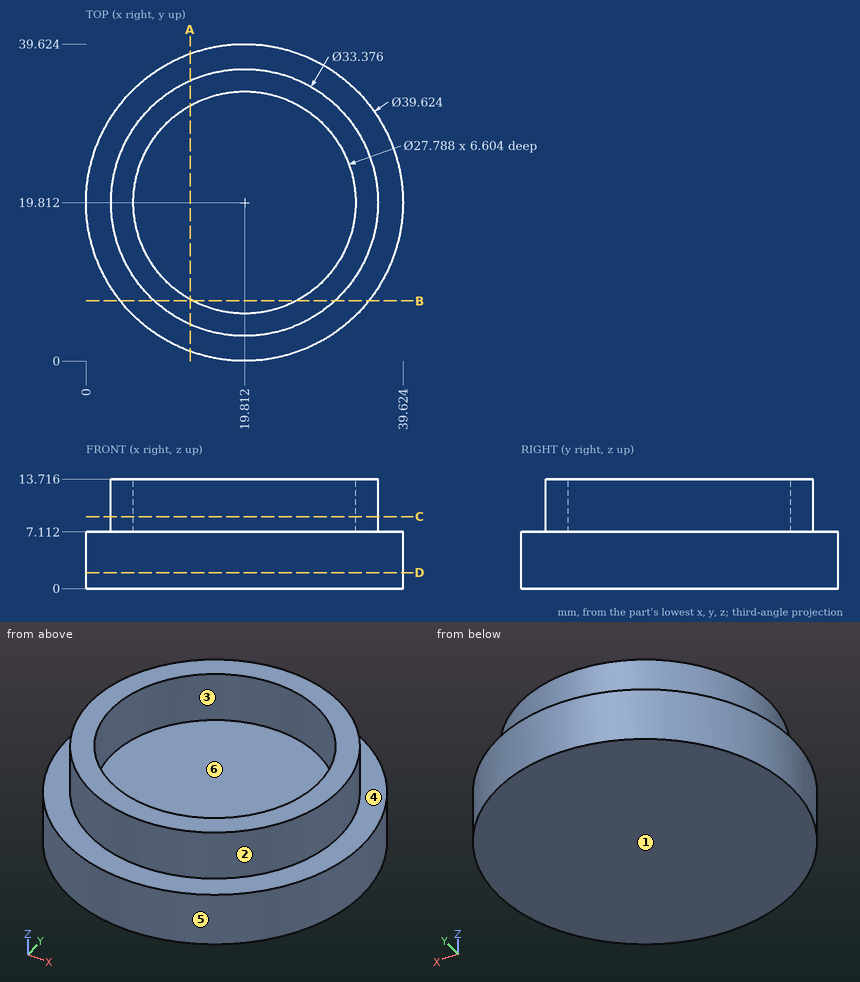
Geometry: see drawing. Coordinates: mm, zero at the bounding-box minimum. A direction names the side the tool comes from. Round coordinates to 2 decimals unless told otherwise and drop trailing zeros. Loops run counter-clockwise (first coordinate to the right, second up) from the corner with the lowest first, then second, coordinate; pieces in that order, holes last.
(1) Section query A-A (x = 13). Output: boundary loops of the cut face in (y, z), and give its area (3 significant figures).
From the geometry:
outline: (1.21, 0) - (38.42, 0) - (38.42, 7.11) - (35.05, 7.11) - (35.05, 13.72) - (31.92, 13.72) - (31.92, 7.11) - (7.7, 7.11) - (7.7, 13.72) - (4.58, 13.72) - (4.58, 7.11) - (1.21, 7.11) - close
area: 306 mm2
(2) Section query C-C (z = 9). Output: boundary loops of the cut face in (x, y) (1 decimal).
From the geometry:
outline: circle Ø33.4 at (19.8, 19.8); hole circle Ø27.8 at (19.8, 19.8)
(3) Material intervals for probe 1 along Y at (x, z) = (25.5, 9.25) (1 decimal); probe 2 along X at (y, z) = (19.5, 2); probe 3 along Z at (x, y) = (15, 17.5), sorted ascending.
From the geometry:
probe 1: y = 4.1 to 7.1, 32.5 to 35.5
probe 2: x = 0 to 39.62
probe 3: z = 0 to 7.11
(4) Access query for the marked faces 1 and 2. Directions: +Z, -Z, +X, -X, +Y, -Y. A direction counts if a zero-diameter tool reaches every point of the face in a straight line with its end or side. Return the directions, or none.
From the geometry:
face 1: -Z, +X, -X, +Y, -Y
face 2: +Z
(5) Pull-direction query (Y, two-part tool) for the marked faces 3, 4, 5 and 6; classes: +Y half, -Y half, draft (parallel to the pull), parting line (faces both ways), or undercut.
From the geometry:
face 3: undercut
face 4: draft
face 5: parting line
face 6: undercut
(6) Contact query for flat-ended pins moving along their axis: pin 1 Ø3 at (y, z) = (18, 4.5) entering from +X; pin 2 Ø5 at (x, z) = (34.5, 12) entering from +Y; pin 3 Ø5 at (x, z) = (10.5, 8) entering from +Y (1 decimal). Output: stop coordinate, or through.
From the geometry:
pin 1: stops at x = 39.62
pin 2: stops at y = 31.21
pin 3: stops at y = 38.4
(7) Section query B-B (y = 7.5). Output: boundary loops of the cut face in (x, z).
From the geometry:
outline: (4.29, 0) - (35.33, 0) - (35.33, 7.11) - (31.08, 7.11) - (31.08, 13.72) - (26.25, 13.72) - (26.25, 7.11) - (13.37, 7.11) - (13.37, 13.72) - (8.55, 13.72) - (8.55, 7.11) - (4.29, 7.11) - close
(8) Section query D-D (z = 2). Output: boundary loops of the cut face in (x, y).
From the geometry:
outline: circle Ø39.62 at (19.81, 19.81)
